```python
from build123d import *

# Parameters (mm, degrees)
F0_R      = 6.75
F1_DEPTH  = 1.5
F2_R      = 4.575
F3_DEPTH  = 9.05
F4_R      = 3.85
F5_DEPTH  = 3.25
F6_SIZE2  = 1
F6_SIZE   = 0.5
F7_R      = 3.35
F8_DEPTH  = 1.5
F9_R      = 4.25
F10_DEPTH = 3.25
F11_R     = 1.75


with BuildPart() as f1:
    # F0 (on Top) → F1 (new body)
    with BuildSketch(Plane.XY):
        Circle(F0_R)
    extrude(amount=F1_DEPTH)

    # F2 (on face) → F3 (join)
    with BuildSketch(Plane(origin=(0, 0, 0), x_dir=(1, 0, 0), z_dir=(0, 0, -1))):
        Circle(F2_R)
    extrude(amount=F3_DEPTH)

    # F4 (on face) → F5 (join)
    with BuildSketch(Plane(origin=(0, 0, -9.05), x_dir=(1, 0, 0), z_dir=(0, 0, -1))):
        Circle(F4_R)
    extrude(amount=F5_DEPTH)

    # F6
    f6_edges = [f1.edges().sort_by_distance(p)[0] for p in [
        (-3.85, 0, -12.3),
    ]]
    f6_side = f1.faces().sort_by_distance((0, 0, -12.3))[0]
    chamfer(f6_edges, length=F6_SIZE, length2=F6_SIZE2, reference=f6_side)

    # F7 (on face) → F8 (join)
    with BuildSketch(Plane(origin=(0, 0, -12.3), x_dir=(1, 0, 0), z_dir=(0, 0, -1))):
        Circle(F7_R)
    extrude(amount=F8_DEPTH)

    # F9 (on face) → F10 (join)
    with BuildSketch(Plane(origin=(0, 0, -13.8), x_dir=(1, 0, 0), z_dir=(0, 0, -1))):
        Circle(F9_R)
    extrude(amount=F10_DEPTH)

    # F11
    f11_edges = [f1.edges().sort_by_distance(p)[0] for p in [
        (-4.25, 0, -17.05),
    ]]
    fillet(f11_edges, radius=F11_R)


solid = f1.part
```
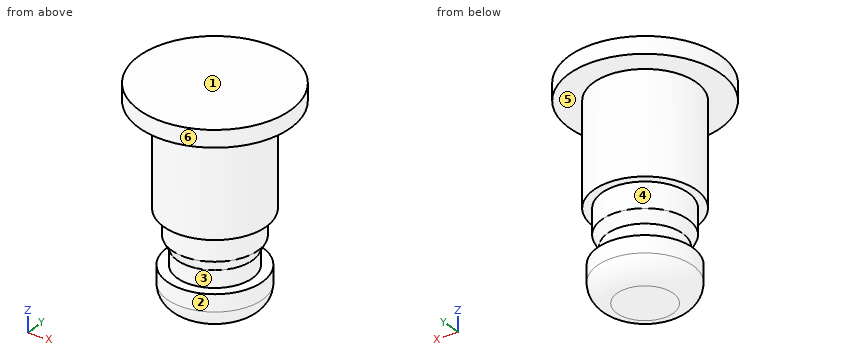
The listing builds one solid part. Answer for the finished solid, in the listing's coordinates (mm). Face numbers are marked on the shaded views. A direction names the side the tool comes from. Coordinates: 2 decimals unless noted, no trailing zeros. Loops run counter-clockwise (first coordinate to the right, second up) from the corner with the lowest first, then second, coordinate; pieces in that order, holes last. Notation, with made-up numbers: (24.5, 52.5) -> (59.5, 52.5) arc R16 cw to (59.5, 73.5) -> close; hole circle Ø6 at (65, 40.25). An arc over 180 degrees is marked (long way). Return JSON: item names as keys, results as strings. Group by question number.
(1) Find the intervals of material crossed by probe 1 along Z at (x, y) = (1.5, 4.75); probe 2 along Y at (x, z) = (0, -13); probe 3 along Z at (x, y) = (3.5, 2.75), in increasing order. Write a range as from..to.
(2) Determine the mould class of the marked faces 3, 4, 5 and 6 for opening direction Z: released by +Z, released by -Z, zero draft, split by the parting line, or undercut.
(3) Given pin 1 Ø4 at (x, z) = (0.5, -5) entering from -Y (3 decimals); pin 2 Ø8 at (x, z) = (3.5, -3) entering from +Y; pin 3 Ø6 at (y, z) = (-3, -5) entering from -X (3 decimals), each flat-ended and moving along its own axis, determine where each tip first touches the part or whether it passes through.
(4) A cutting plane is placed at A-A on y = 0. Write down the section's boundary in (x, z) (3 decimals), and give its area (3 significant figures).
(5) A cutting plane is placed at C-C on z = -14.25. Write down the section's boundary in (x, y).
(6) Which of the six approach directions +Z, -Z, +X, -X, +Y, -Y give full straight-line access (tool end or side, diameter ignored) to the marked faces 1 and 2?
(7) A cutting plane is placed at D-D on z = -3.5. Write down the section's boundary in (x, y) (3 decimals).
The answers:
{
 "1": {"probe 1": "z = 0..1.5", "probe 2": "y = -3.35..3.35", "probe 3": "z = -9.05..1.5"},
 "2": {"face 3": "undercut", "face 4": "undercut", "face 5": "released by -Z", "face 6": "zero draft"},
 "3": {"pin 1": "stops at y = -4.575", "pin 2": "stops at y = 6.7", "pin 3": "stops at x = -4.575"},
 "4": {"outline": "(-6.75, 0) -> (-4.575, 0) -> (-4.575, -9.05) -> (-3.85, -9.05) -> (-3.85, -11.3) -> (-3.35, -12.3) -> (-3.35, -13.8) -> (-4.25, -13.8) -> (-4.25, -15.3) arc R1.75 ccw to (-2.5, -17.05) -> (2.5, -17.05) arc R1.75 ccw to (4.25, -15.3) -> (4.25, -13.8) -> (3.35, -13.8) -> (3.35, -12.3) -> (3.85, -11.3) -> (3.85, -9.05) -> (4.575, -9.05) -> (4.575, 0) -> (6.75, 0) -> (6.75, 1.5) -> (-6.75, 1.5) -> close", "area": "164 mm^2"},
 "5": {"outline": "circle Ø8.5 at (0, 0)"},
 "6": {"face 1": "+Z, +X, -X, +Y, -Y", "face 2": "-Z"},
 "7": {"outline": "circle Ø9.15 at (0, 0)"}
}
